from build123d import *

# Parameters (mm, degrees)
SKETCH1_R           = 1.65
BOSS_EXTRUDE1_DEPTH = 7.6
CUT_EXTRUDE1_REACH  = 89.547
SKETCH3_W           = 6.5
SKETCH3_H           = 15.5
SKETCH3_H_2         = 14
SKETCH3_H_3         = 16.6
CUT_EXTRUDE2_DEPTH  = 3.3
FILLET1_R           = 3


with BuildPart() as part:
    # Sketch1 → Boss-Extrude1 (new body)
    with BuildSketch(Plane.XY):
        Polygon((19.2, 59.55), (19.2, 8.85), (32.2, 8.85), (32.2, -3.15), (40.2, -3.15), (40.2, -77.4), (-40.2, -77.4), (-40.2, -3.15), (-32.2, -3.15), (-32.2, 8.85), (-19.2, 8.85), (-19.2, 59.55), align=None)
        with Locations((29.2, 5.85)):
            Circle(SKETCH1_R, mode=Mode.SUBTRACT)
        with Locations((29.2, -0.15)):
            Circle(SKETCH1_R, mode=Mode.SUBTRACT)
        with Locations((37.2, -55.4)):
            Circle(SKETCH1_R, mode=Mode.SUBTRACT)
        with Locations((37.2, -64)):
            Circle(SKETCH1_R, mode=Mode.SUBTRACT)
        with Locations((16.2, 48.05)):
            Circle(SKETCH1_R, mode=Mode.SUBTRACT)
        with Locations((16.2, 54.55)):
            Circle(SKETCH1_R, mode=Mode.SUBTRACT)
        with Locations(Location((-16.2, 54.55, 0), (0, 0, 180))):
            Circle(SKETCH1_R, mode=Mode.SUBTRACT)
        with Locations(Location((-16.2, 48.05, 0), (0, 0, 180))):
            Circle(SKETCH1_R, mode=Mode.SUBTRACT)
        with Locations(Location((-37.2, -64, 0), (0, 0, 180))):
            Circle(SKETCH1_R, mode=Mode.SUBTRACT)
        with Locations(Location((-37.2, -55.4, 0), (0, 0, 180))):
            Circle(SKETCH1_R, mode=Mode.SUBTRACT)
        with Locations(Location((-29.2, -0.15, 0), (0, 0, 180))):
            Circle(SKETCH1_R, mode=Mode.SUBTRACT)
        with Locations(Location((-29.2, 5.85, 0), (0, 0, 180))):
            Circle(SKETCH1_R, mode=Mode.SUBTRACT)
    extrude(amount=-BOSS_EXTRUDE1_DEPTH)

    # Sketch2 → Cut-Extrude1 (cut, up to next)
    with BuildSketch(Plane(origin=(0, 0, -7.6), x_dir=(-1, 0, 0), z_dir=(0, 0, -1)), mode=Mode.PRIVATE) as cut_extrude1_sk1:
        Polygon((-12.7, 2.35), (-12.7, 53.05), (12.7, 53.05), (12.7, 2.35), (25.7, 2.35), (25.7, -9.65), (33.7, -9.65), (33.7, -70.9), (40.2, -70.9), (40.2, -77.4), (-40.2, -77.4), (-40.2, -70.9), (-33.7, -70.9), (-33.7, -9.65), (-25.7, -9.65), (-25.7, 2.35), align=None)
    cut_extrude1_tool1 = extrude(cut_extrude1_sk1.sketch, amount=-CUT_EXTRUDE1_REACH, mode=Mode.PRIVATE) & part.part
    add(cut_extrude1_tool1.solids().sort_by_distance((0, -26.176143, -7.6))[0], mode=Mode.SUBTRACT)

    # Sketch3 → Cut-Extrude2 (cut)
    with BuildSketch(Plane(origin=(0, 0, 0), x_dir=(-1, 0, 0), z_dir=(0, 0, -1))):
        with Locations((15.95, 51.8)):
            Rectangle(SKETCH3_W, SKETCH3_H)
        with Locations((28.95, 2.85)):
            Rectangle(SKETCH3_W, SKETCH3_H_2)
        with Locations((36.95, -59.7)):
            Rectangle(SKETCH3_W, SKETCH3_H_3)
    cut_extrude2 = extrude(amount=CUT_EXTRUDE2_DEPTH, mode=Mode.SUBTRACT)

    # Mirror1: Cut-Extrude2 across plane
    add(cut_extrude2.mirror(Plane(origin=(0, 0, 0), x_dir=(0, 0, 1), z_dir=(1, 0, 0))), mode=Mode.SUBTRACT)

    # Fillet1
    fillet1_edges = [part.edges().sort_by_distance(p)[0] for p in [
        (-25.7, 2.35, -5.45),
        (-12.7, 53.05, -5.45),
        (19.2, 8.85, -3.8),
        (32.2, -3.15, -5.45),
        (25.7, 2.35, -5.45),
        (12.7, 53.05, -5.45),
        (-32.2, -3.15, -5.45),
        (-19.2, 8.85, -3.8),
        (-33.7, -9.65, -3.8),
        (33.7, -9.65, -3.8),
    ]]
    fillet(fillet1_edges, radius=FILLET1_R)


solid = part.part
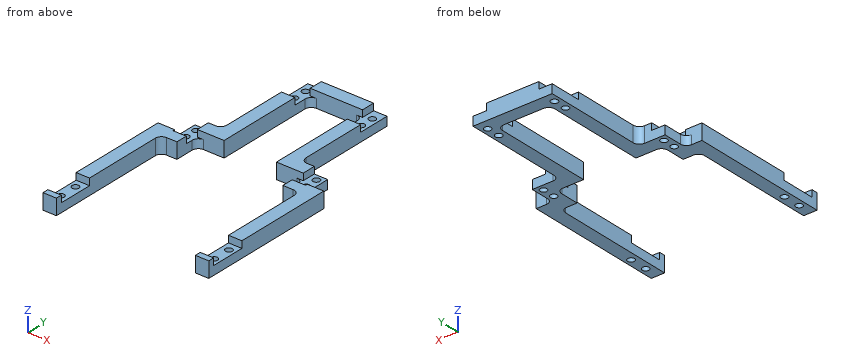
Could you check a few things on this model? Use its own coordinates, in mm. Coordinates: 2 decimals unless noted, no trailing zeros. Order: outer loops, then holes, each group sorted by start corner. A loop starts at its lowest first (then second) coordinate and runs counter-clockwise, first axis right, second up. Notation, with made-up numbers: (1.5, 87.5) - (53.5, 87.5) arc R31 cw to (53.5, 118.5) - close; hole circle Ø5 at (23.25, -20). An arc over 180 degrees is marked (long way). Answer in a Markdown table with one row per item. Add a question column.
(1) I need wall thicknesses on L1, parallel to Y at x = -16.2, z = -4.95; L2, parallel to Y at x = 37.2, z = -5; L3, parallel to X at y = -25, z = -2.75. Which ranges of each line are inside material? Lowest first, please.
(2) If we section it at A-A, the plane y = -32: Please give me the cut outline in (x, z), then the cut area to 3 significant figures.
(3) If we section it at D-D, the plane y = 54.55: Please give me the cut outline in (x, z).
(4) If we section it at C-C, the plane y = -55.4: Please give me the cut outline in (x, z).
(5) Will these pins go through, and if not, where does the flat tip stop? pin 1 (4 mm diameter, centred on x = 19.5, z = -5.5, fed in from -Y); pin 2 (3 mm diameter, centred on y = 42, z = -6, fed in from -X); pin 3 (4.5 mm diameter, centred on x = 37.2, y = -55.4, fed in from +Z); pin 4 (2.5 mm diameter, centred on x = -29.2, y = -0.15, fed in from -Z).
(6) If we section it at B-B, the plane x = -29.2: Please give me the cut outline in (y, z).
Results are:
| question | item | result |
|---|---|---|
| 1 | L1 | y = 2.35 to 46.4, 49.7 to 52.9, 56.2 to 59.55 |
| 1 | L2 | y = -70.9 to -65.65, -62.35 to -57.05, -53.75 to -3.15 |
| 1 | L3 | x = -40.2 to -33.7, 33.7 to 40.2 |
| 2 | outline | (-40.2, -7.6) - (-33.7, -7.6) - (-33.7, 0) - (-40.2, 0) - close; (33.7, -7.6) - (40.2, -7.6) - (40.2, 0) - (33.7, 0) - close |
| 2 | area | 98.8 mm2 |
| 3 | outline | (-19.2, -7.6) - (-17.85, -7.6) - (-17.85, -3.3) - (-19.2, -3.3) - close; (-14.55, -7.6) - (14.55, -7.6) - (14.55, -3.3) - (12.7, -3.3) - (12.7, 0) - (-12.7, 0) - (-12.7, -3.3) - (-14.55, -3.3) - close; (17.85, -7.6) - (19.2, -7.6) - (19.2, -3.3) - (17.85, -3.3) - close |
| 4 | outline | (-40.2, -7.6) - (-38.85, -7.6) - (-38.85, -3.3) - (-40.2, -3.3) - close; (-35.55, -7.6) - (-33.7, -7.6) - (-33.7, -3.3) - (-35.55, -3.3) - close; (33.7, -7.6) - (35.55, -7.6) - (35.55, -3.3) - (33.7, -3.3) - close; (38.85, -7.6) - (40.2, -7.6) - (40.2, -3.3) - (38.85, -3.3) - close |
| 5 | pin 1 | stops at y = 2.35 |
| 5 | pin 2 | stops at x = -19.2 |
| 5 | pin 3 | stops at z = -3.3 |
| 5 | pin 4 | passes through |
| 6 | outline | (-9.65, -7.6) - (-1.8, -7.6) - (-1.8, -3.3) - (-4.15, -3.3) - (-4.15, 0) - (-9.65, 0) - close; (1.5, -7.6) - (4.2, -7.6) - (4.2, -3.3) - (1.5, -3.3) - close; (7.5, -7.6) - (8.85, -7.6) - (8.85, -3.3) - (7.5, -3.3) - close |
